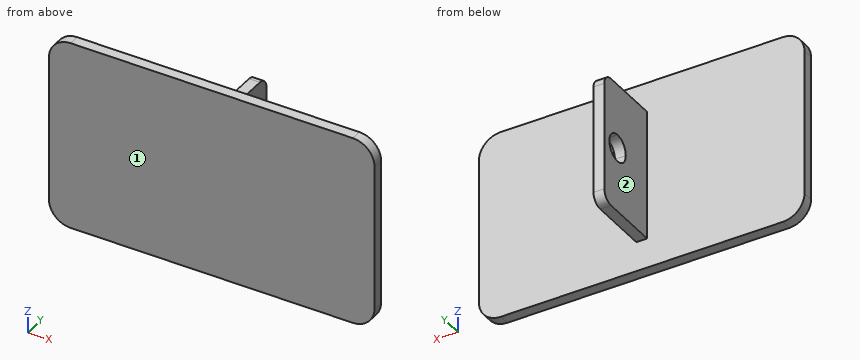
from build123d import *

# Parameters (mm, degrees)
SKETCH1_W           = 300
SKETCH1_H           = 175
BOSS_EXTRUDE1_DEPTH = 10
SKETCH2_W           = 10
SKETCH2_H           = 120
BOSS_EXTRUDE2_DEPTH = 65
CUT_EXTRUDE1_DEPTH  = 10
FILLET1_R           = 10
FILLET2_R           = 20


with BuildPart() as part:
    # Sketch1 → Boss-Extrude1 (new body)
    with BuildSketch(Plane(origin=(0, 0, 0), x_dir=(1, 0, 0), z_dir=(0, 1, 0))):
        Rectangle(SKETCH1_W, SKETCH1_H)
    extrude(amount=BOSS_EXTRUDE1_DEPTH)

    # Sketch2 → Boss-Extrude2 (add)
    with BuildSketch(Plane(origin=(0, 10, 0), x_dir=(1, 0, 0), z_dir=(0, 1, 0))):
        Rectangle(SKETCH2_W, SKETCH2_H)
    extrude(amount=BOSS_EXTRUDE2_DEPTH)

    # Sketch3 → Cut-Extrude1 (cut)
    with BuildSketch(Plane(origin=(5, 0, 0), x_dir=(0, 0, -1), z_dir=(1, 0, 0))):
        with BuildLine():
            ThreePointArc((-12.5, 55), (-8.838834765, 46.161165235), (0, 42.5))
            Line((0, 42.5), (0, 55))
            Line((0, 55), (-12.5, 55))
        make_face()
        with BuildLine():
            Line((0, 55), (0, 42.5))
            ThreePointArc((0, 42.5), (8.838834765, 46.161165235), (12.5, 55))
            Line((12.5, 55), (0, 55))
        make_face()
        with BuildLine():
            Line((-12.5, 55), (0, 55))
            Line((0, 55), (12.5, 55))
            ThreePointArc((12.5, 55), (0, 67.5), (-12.5, 55))
        make_face()
    extrude(amount=-CUT_EXTRUDE1_DEPTH, mode=Mode.SUBTRACT)

    # Fillet1
    fillet1_edges = [part.edges().sort_by_distance(p)[0] for p in [
        (0, 75, -60),
        (0, 75, 60),
    ]]
    fillet(fillet1_edges, radius=FILLET1_R)

    # Fillet2
    fillet2_edges = [part.edges().sort_by_distance(p)[0] for p in [
        (150, 5, 87.5),
        (-150, 5, 87.5),
        (-150, 5, -87.5),
        (150, 5, -87.5),
    ]]
    fillet(fillet2_edges, radius=FILLET2_R)


solid = part.part
The listing builds one solid part. Answer for the finished solid, in the listing's coordinates (mm). Face numbers are marked on the shaded views. A direction names the side the tool comes from. Give positions to 0.01 mm unless a question says otherwise; leave off trailing zeros. Loops run counter-clockwise (first coordinate to the right, second up) from the corner with the lowest first, then second, coordinate; pieces in that order, holes last. Notation, with made-up numbers: (74, 17) - (88, 17) arc R31 ccw to (88, 46) - close; hole circle Ø2 at (64.25, 63). An arc over 180 degrees is marked (long way). Answer as a JSON object with one key per item and string values.
1. For the marked faces 1 and 2, determine the directions among +Z, -Z, +X, -X, +Y, -Y from which every point of the face is accessible in a straight line to the end or side of a thin tool.
Determined:
{"face 1": "+Z, -Z, +X, -X, -Y", "face 2": "+Z, -Z, -X, +Y"}
2. A cutting plane is placed at A-A (y = 49). Write down the section's boundary in (x, z).
Determined:
{"outline": "(-5, -60) - (5, -60) - (5, -10.97) - (-5, -10.97) - close; (-5, 10.97) - (5, 10.97) - (5, 60) - (-5, 60) - close"}
3. A cutting plane is placed at D-D (y = 32.5). Write down the section's boundary in (x, z).
Determined:
{"outline": "(-5, -60) - (5, -60) - (5, 60) - (-5, 60) - close"}
4. Find the intervals of material crossed by L1, parallel to X at y = 40.5, z = -51; L2, parallel to Y at x = 129, z = -74; L3, parallel to Z at x = 4, y = 36, in increasing order. Write a range as [from, to].
Determined:
{"L1": "[-5, 5]", "L2": "[0, 10]", "L3": "[-60, 60]"}
5. A cutting plane is placed at C-C (x = 115). Write down the section's boundary in (y, z), then the cut area to 3 significant figures.
Determined:
{"outline": "(0, -87.5) - (10, -87.5) - (10, 87.5) - (0, 87.5) - close", "area": "1,750 mm²"}
6. A cutting plane is placed at B-B (z = 55.5). Write down the section's boundary in (x, y), then the cut area to 3 significant figures.
Determined:
{"outline": "(-150, 0) - (150, 0) - (150, 10) - (5, 10) - (5, 73.35) - (-5, 73.35) - (-5, 10) - (-150, 10) - close", "area": "3,630 mm²"}
7. Flat-ended cylindrical pins translate along their axes: pin 1 Ø1 at (y, z) = (50.5, 24) entering from -X; pin 2 Ø8 at (x, y) = (2, 29) entering from +Z; pin 3 Ø8 at (x, y) = (2, 25) entering from -Z. Find the tip coordinate at first contact, or state that the pin passes through.
Determined:
{"pin 1": "x = -5", "pin 2": "z = 60", "pin 3": "z = -60"}
